from build123d import *

# Parameters (mm, degrees)
SKETCH1_W           = 7.8
SKETCH1_H           = 3.2
BOSS_EXTRUDE1_DEPTH = 7.8
SKETCH2_R           = 2.4
BOSS_EXTRUDE2_DEPTH = 1.6
SKETCH3_W           = 6.5
SKETCH3_H           = 5.4
CUT_EXTRUDE1_DEPTH  = 3
SKETCH4_R           = 1.3
CUT_EXTRUDE2_DEPTH  = 1.7
SKETCH5_W           = 7.8
SKETCH5_H           = 7.134621369
BOSS_EXTRUDE3_DEPTH = 1.4
FILLET1_R           = 0.5
SKETCH6_R           = 1.75
SKETCH6_R_2         = 1.05
BOSS_EXTRUDE4_DEPTH = 1.5


with BuildPart() as part:
    # Sketch1 → Boss-Extrude1 (new body)
    with BuildSketch(Plane.XY):
        with Locations((3.9, 1.6)):
            Rectangle(SKETCH1_W, SKETCH1_H)
    extrude(amount=-BOSS_EXTRUDE1_DEPTH)

    # Sketch2 → Boss-Extrude2 (add)
    with BuildSketch(Plane(origin=(0, 3.2, 0), x_dir=(1, 0, 0), z_dir=(0, 1, 0))):
        with Locations(Location((3.9, 3.9, 0), (0, 0, 270))):
            Circle(SKETCH2_R)
    extrude(amount=BOSS_EXTRUDE2_DEPTH)

    # Sketch3 → Cut-Extrude1 (cut)
    with BuildSketch(Plane.XZ):
        with Locations((4.45, -3.9)):
            Rectangle(SKETCH3_W, SKETCH3_H)
    extrude(amount=-CUT_EXTRUDE1_DEPTH, mode=Mode.SUBTRACT)

    # Sketch4 → Cut-Extrude2 (cut)
    with BuildSketch(Plane.XZ.offset(-3)):
        with Locations(Location((3.9, -3.9, 0), (0, 0, 270))):
            Circle(SKETCH4_R)
    extrude(amount=-CUT_EXTRUDE2_DEPTH, mode=Mode.SUBTRACT)

    # Sketch5 → Boss-Extrude3 (add)
    with BuildSketch(Plane(origin=(7.8, 0, 0), x_dir=(0, 0, -1), z_dir=(1, 0, 0))):
        with Locations((3.9, 3.567310685)):
            Rectangle(SKETCH5_W, SKETCH5_H)
    extrude(amount=BOSS_EXTRUDE3_DEPTH)

    # Fillet1
    fillet1_edges = [part.edges().sort_by_distance(p)[0] for p in [
        (8.5, 7.134621369, -7.8),
        (8.5, 7.134621369, 0),
    ]]
    fillet(fillet1_edges, radius=FILLET1_R)

    # Sketch6 → Boss-Extrude4 (add)
    with BuildSketch(Plane(origin=(9.2, 0, 0), x_dir=(0, 0, -1), z_dir=(1, 0, 0))):
        with Locations(Location((3.9, 4.134621369, 0), (0, 0, 180))):
            Circle(SKETCH6_R)
        with Locations((3.9, 4.134621369)):
            Circle(SKETCH6_R_2, mode=Mode.SUBTRACT)
    extrude(amount=BOSS_EXTRUDE4_DEPTH)


solid = part.part
Verification items for the finished model (mm, model axes). A direction names the side the tool comes from. Give positions to 0.01 mm unless a question says otherwise; leave off trailing zeros. Write each loop counter-clockwise with the first axis right and the second up, starting at its lowest first coordinate (ties: lowest second). Pieces come first, ordered by that corner, then holes. Notation, with made-up numbers: M 48.5,64.5 L 71.5,64.5 A23 ccw 71.5,88.5 Z; hole C -37.75,0.25 d3. An arc over 180 degrees is marked long. Put each result on its own line as item: value. Start each with the question number.
1. Set-up check for faces 1 (the face through (2, 3.2, -2)), 2 (the face through (9.939, 5.843, -4.279)), 3 (the face through (4, 1, -6.6)): record each of +Z, -Z, +X, -X, +Y, -Y from which the full face is reachable in a straight line by a thin tool's end or side.
2. Section check A-A (y = 4). Record the cut outline in (x, z).
3. Go/stop test with flat-tipped pins: pin 1 Ø1.5 at (x, z) = (7, -1) entering from +Y; pin 2 Ø4 at (x, z) = (3.9, -3.9) entering from +Y; pin 3 Ø2 at (x, z) = (4, -3.5) entering from -Y. Record where each tip stops, or that it passes through.
4. Section check B-B (z = -3.9). Record the cut outline in (x, y).
5. Section check C-C (x = 7). Record the cut outline in (y, z).
6. Scan lines: line 1 along X through (y, z) = (3.8, -3.9); line 2 along Y through (x, z) = (9.85, -3.9); line 3 along Z through (x, y) = (6.25, 2.5). Record each from-to range of solid material in increasing order. Write a range as [from, to].
7. Draft check along X on faces 4 (the face through (5, 2, 0)), 5 (the face through (10.7, 5, -3)), 6 (the face through (7.8, 5, -4)). Enter one of: +X half, -X half, draft (parallel to the pull), parting line (faces both ways), or undercut.
8. Section check D-D (y = 0.5). Record the cut outline in (x, z).
Answer list:
1. face 1: +Y
1. face 2: +X
1. face 3: -Y
2. outline: C 3.9,-3.9 d4.8; M 7.8,-7.8 L 9.2,-7.8 L 9.2,-5.64 L 10.7,-5.64 L 10.7,-4.94 L 9.2,-4.94 L 9.2,-2.86 L 10.7,-2.86 L 10.7,-2.16 L 9.2,-2.16 L 9.2,0 L 7.8,0 Z; hole C 3.9,-3.9 d2.6
3. pin 1: y = 3.2
3. pin 2: y = 4.8
3. pin 3: y = 3
4. outline: M 0,0 L 1.2,0 L 1.2,3 L 2.6,3 L 2.6,4.7 L 5.2,4.7 L 5.2,3 L 7.7,3 L 7.7,0 L 9.2,0 L 9.2,2.38 L 10.7,2.38 L 10.7,3.08 L 9.2,3.08 L 9.2,5.18 L 10.7,5.18 L 10.7,5.88 L 9.2,5.88 L 9.2,7.13 L 7.8,7.13 L 7.8,3.2 L 6.3,3.2 L 6.3,4.8 L 1.5,4.8 L 1.5,3.2 L 0,3.2 Z
5. outline: M 0,-7.8 L 3.2,-7.8 L 3.2,0 L 0,0 L 0,-1.2 L 3,-1.2 L 3,-6.6 L 0,-6.6 Z
6. line 1: [1.5, 2.6], [5.2, 6.3], [7.8, 9.2]
6. line 2: [2.38, 3.08], [5.18, 5.88]
6. line 3: [-7.8, -6.6], [-1.2, 0]
7. face 4: draft
7. face 5: +X half
7. face 6: undercut
8. outline: M 0,-7.8 L 9.2,-7.8 L 9.2,0 L 0,0 Z; hole M 1.2,-6.6 L 7.7,-6.6 L 7.7,-1.2 L 1.2,-1.2 Z
